from build123d import *

# Parameters (mm, degrees)
SKETCH2_W           = 16.5
SKETCH2_H           = 40
BOSS_EXTRUDE1_DEPTH = 20
CUT_EXTRUDE1_DEPTH  = 20
SKETCH5_W           = 46.207326837
SKETCH5_H           = 41.881023155
CUT_EXTRUDE2_DEPTH  = 20
SKETCH1_R           = 2.1
CUT_EXTRUDE3_DEPTH  = 5.7
SKETCH7_R           = 2.1
CUT_EXTRUDE4_DEPTH  = 5.7


with BuildPart() as part:
    # Sketch2 → Boss-Extrude1 (new body)
    with BuildSketch(Plane(origin=(0, 20, 0), x_dir=(1, 0, 0), z_dir=(0, 1, 0))):
        with Locations((-8.25, 0)):
            Rectangle(SKETCH2_W, SKETCH2_H)
        with Locations((8.25, 0)):
            Rectangle(SKETCH2_W, SKETCH2_H)
    extrude(amount=-BOSS_EXTRUDE1_DEPTH)

    # Sketch4 → Cut-Extrude1 (cut)
    with BuildSketch(Plane(origin=(9.044657999, -2.93951385, 0), x_dir=(0, 0, 1), z_dir=(-0.9510340687309481, 0.30908607233755875, 0))):
        Polygon((-21.945163579, 1.558302269), (-22.817048797, 25.42042402), (26.491055296, 25.42042402), (24.942749687, 1.558302269), align=None)
    cut_extrude1 = extrude(amount=-CUT_EXTRUDE1_DEPTH, mode=Mode.SUBTRACT)

    # Sketch5 → Cut-Extrude2 (cut)
    with BuildSketch(Plane(origin=(0, -4, -8), x_dir=(1, 0, 0), z_dir=(0, 0.447213595499958, 0.894427190999916))):
        with Locations((1.743983375, 9.495933816)):
            Rectangle(SKETCH5_W, SKETCH5_H)
    cut_extrude2 = extrude(amount=-CUT_EXTRUDE2_DEPTH, mode=Mode.SUBTRACT)

    # Mirror1: Cut-Extrude2 across plane
    add(cut_extrude2.mirror(Plane.XY), mode=Mode.SUBTRACT)

    # Mirror2: Cut-Extrude1 across plane
    add(cut_extrude1.mirror(Plane(origin=(0, 0, 0), x_dir=(0, 0, 1), z_dir=(1, 0, 0))), mode=Mode.SUBTRACT)

    # Sketch1 → Cut-Extrude3 (cut)
    with BuildSketch(Plane(origin=(0, 0, 0), x_dir=(1, 0, 0), z_dir=(0, 1, 0))):
        with Locations(Location((-5, 5, 0), (0, 0, 270))):
            Circle(SKETCH1_R)
        with Locations(Location((5, 5, 0), (0, 0, 270))):
            Circle(SKETCH1_R)
        with Locations(Location((5, -5, 0), (0, 0, 270))):
            Circle(SKETCH1_R)
        with Locations(Location((-5, -5, 0), (0, 0, 270))):
            Circle(SKETCH1_R)
    extrude(amount=CUT_EXTRUDE3_DEPTH, mode=Mode.SUBTRACT)

    # Sketch7 → Cut-Extrude4 (cut)
    with BuildSketch(Plane(origin=(0, 20, 0), x_dir=(1, 0, 0), z_dir=(0, 1, 0))):
        with Locations(Location((-11.5, 15, 0), (0, 0, 270))):
            Circle(SKETCH7_R)
        with Locations(Location((-11.5, -15, 0), (0, 0, 90))):
            Circle(SKETCH7_R)
        with Locations(Location((11.5, -15, 0), (0, 0, 270))):
            Circle(SKETCH7_R)
        with Locations(Location((11.5, 15, 0), (0, 0, 90))):
            Circle(SKETCH7_R)
    extrude(amount=-CUT_EXTRUDE4_DEPTH, mode=Mode.SUBTRACT)


solid = part.part
Model file for the job. Use its own axes, mm. A direction names the side the tool comes from. Give positions to 0.01 mm unless a question says otherwise; leave off trailing zeros. Write each loop counter-clockwise with the first axis right and the second up, starting at its lowest first coordinate (ties: lowest second). Pieces come first, ordered by that corner, then holes. Notation, with made-up numbers: (54.25, -2.5) -> (66.25, -2.5) arc R16 cw to (66.25, 24.5) -> close; hole circle Ø3 at (53.25, -26). An arc over 180 degrees is marked (long way). Write item = value, one per line.
(1) Slice it at C-C, the plane y = 12. Give the cut face in (x, z).
Determined:
outline = (-13.9, -16) -> (13.9, -16) -> (13.9, 16) -> (-13.9, 16) -> close
(2) Probe line 1 along X through (y, z) = (3.5, -3.5); line 2 along X through (y, z) = (18.25, 15); line 3 along Z through (x, y) = (-0.5, 13). List the from-to ranges inside material, lowest first.
Determined:
line_1 = -11.14 to -6.47, -3.53 to 3.53, 6.47 to 11.14
line_2 = -15.93 to -13.6, -9.4 to 9.4, 13.6 to 15.93
line_3 = -16.5 to 16.5
(3) Slice it at A-A, the plane x = 5. Give the cut face in (y, z), then the cut area to 3 significant figures.
Determined:
outline = (0, -10) -> (20, -20) -> (20, 20) -> (0, 10) -> (0, 7.1) -> (5.7, 7.1) -> (5.7, 2.9) -> (0, 2.9) -> (0, -2.9) -> (5.7, -2.9) -> (5.7, -7.1) -> (0, -7.1) -> close
area = 552 mm2
(4) Slice it at B-B, the plane z = 5. Give the cut face in (x, y), then the cut area to 3 significant figures.
Determined:
outline = (-16.5, 20) -> (-10, 0) -> (-7.1, 0) -> (-7.1, 5.7) -> (-2.9, 5.7) -> (-2.9, 0) -> (2.9, 0) -> (2.9, 5.7) -> (7.1, 5.7) -> (7.1, 0) -> (10, 0) -> (16.5, 20) -> close
area = 482 mm2
(5) Slice it at D-D, the plane x = 0.5. Give the cut face in (y, z), then the cut area to 3 significant figures.
Determined:
outline = (0, -10) -> (20, -20) -> (20, 20) -> (0, 10) -> close
area = 600 mm2
(6) Mould opens along Z. For faces 4 (the face through (0, 0, 0)), 5 (the face through (0, 10, -15)), 6 (the face through (-7.05, 2.81, 4.54)) say: released by +Z, released by -Z, zero draft, split by the parting line, or undercut.
Determined:
face_4 = zero draft
face_5 = released by -Z
face_6 = undercut
(7) Tool access for faces 1 (the face through (-7.05, 2.81, -5.46)), 2 (the face through (0, 20, 0)), 3 (the face through (9.418, 17.19, -14.727)): list every direction of +Z, -Z, +X, -X, +Y, -Y with a clear straight run to the whole face (end or side of a thin tool).
Determined:
face_1 = -Y
face_2 = +Z, -Z, +X, -X, +Y
face_3 = +Y
(8) Flat gauge pins, fed straight in: P1, Ø2, axis at x = 12, z = -15, coming from the +Y side; P2, Ø3.5, axis at x = 11.5, z = -15, coming from the -Y side; P3, Ø4.5, axis at x = -5.5, z = 4.5, coming from the -Y side; P4, Ø4, axis at x = 2.5, y = 7, coming from the +Z side. Where does each tip first touch, or does it go through?
Determined:
P1 = 14.3
P2 = 6.5
P3 = 0
P4 = 14.5
